Work out the finished part from the listing and answer in its coordinate system (mm). Give positions to 0.01 mm unless a question says otherwise; leave off trailing zeros. Write each loop counter-clockwise with the first axis right and the second up, starting at its lowest first coordinate (ties: lowest second). Pieces come first, ordered by that corner, then holes.
1) Find section B-B (x = -4). Determine the outline of the cut face in (y, z), plus the area to 3 significant figures.
2) Straight lines are drawn through the part: probe 1 along Y at (x, z) = (-60, 46.45); probe 2 along X at (y, z) = (12.75, -47); probe 3 along Z at (x, y) = (-49, 6.75). For each, find the intervals that lie inside material, in ascending order.
3) Find section C-C (z = -20). Determine the outline of the cut face in (x, y).
4) Find section D-D (y = 8.09). Determine the outline of the cut face in (x, z), plus the area to 3 significant figures.
5) Find section A-A (y = 16.5). Determine the outline of the cut face in (x, z), plus the area to 3 significant figures.
6) Given pin 1 Ø6 at (x, y) = (60, 2.5) entering from +Z; pin 2 Ø2 at (y, z) = (21.5, -49) entering from -X; pin 3 Ø2.5 at (x, z) = (-59, 46) entering from +Y; pin 4 Ø10 at (x, y) = (55.5, 24.5) entering from +Z, each flat-ended and moving along its own axis, determine where each tip first touches the part or whether it passes through.
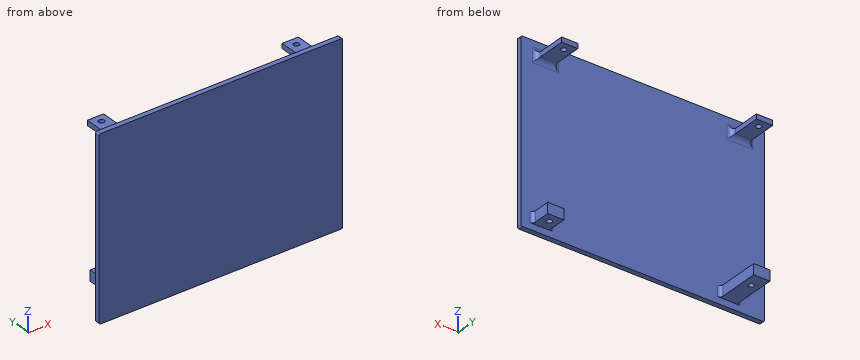
```python
from build123d import *

# Parameters (mm, degrees)
SKETCH1_W            = 150
SKETCH1_H            = 110
BOSS_EXTRUDE1_DEPTH  = 1.5
SKETCH2_W            = 10
SKETCH2_H            = 6.5
BOSS_EXTRUDE2_DEPTH  = 12
SKETCH3_W            = 10
SKETCH3_H            = 6.5
BOSS_EXTRUDE3_DEPTH  = 15
M3_CLEARANCE_HOLE1_D = 3.4
FILLET1_R            = 2
M3_CLEARANCE_HOLE2_D = 3.4
SKETCH8_W            = 10
SKETCH8_H            = 3
BOSS_EXTRUDE4_DEPTH  = 20
FILLET2_R            = 3
M3_CLEARANCE_HOLE3_D = 3.4
FILLET2_OF_MIRROR1_R = 3
FILLET3_R            = 1


with BuildPart() as part:
    # Sketch1 → Boss-Extrude1 (new, symmetric)
    with BuildSketch(Plane(origin=(0, 0, 0), x_dir=(1, 0, 0), z_dir=(0, 1, 0))):
        Rectangle(SKETCH1_W, SKETCH1_H)
    extrude(amount=BOSS_EXTRUDE1_DEPTH, both=True)

    # Sketch2 → Boss-Extrude2 (add)
    with BuildSketch(Plane(origin=(0, 1.5, 0), x_dir=(1, 0, 0), z_dir=(0, 1, 0))):
        with Locations((62.57, 47.75)):
            Rectangle(SKETCH2_W, SKETCH2_H)
        with Locations((-53, 47.75)):
            Rectangle(SKETCH2_W, SKETCH2_H)
    extrude(amount=BOSS_EXTRUDE2_DEPTH)

    # Sketch3 → Boss-Extrude3 (add)
    with BuildSketch(Plane(origin=(0, 13.5, 0), x_dir=(1, 0, 0), z_dir=(0, 1, 0))):
        with Locations((-53, 47.75)):
            Rectangle(SKETCH3_W, SKETCH3_H)
    extrude(amount=BOSS_EXTRUDE3_DEPTH)

    # M3 Clearance Hole1 (through all)
    with Locations(Plane.XY.offset(-44.5)):
        with Locations((-53, 19.77)):
            Hole(M3_CLEARANCE_HOLE1_D / 2)

    # Fillet1
    fillet1_edges = [part.edges().sort_by_distance(p)[0] for p in [
        (67.57, 1.5, -47.75),
        (57.57, 1.5, -47.75),
        (-48, 1.5, -47.75),
        (-58, 1.5, -47.75),
    ]]
    fillet(fillet1_edges, radius=FILLET1_R)

    # M3 Clearance Hole2 (through all)
    with Locations(Plane.XY.offset(-44.5)):
        with Locations((62.57, 8.09)):
            Hole(M3_CLEARANCE_HOLE2_D / 2)

    # Sketch8 → Boss-Extrude4 (add)
    with BuildSketch(Plane(origin=(0, 1.5, 0), x_dir=(1, 0, 0), z_dir=(0, 1, 0))):
        with Locations((-60, -46.5)):
            Rectangle(SKETCH8_W, SKETCH8_H)
    boss_extrude4 = extrude(amount=BOSS_EXTRUDE4_DEPTH)

    # Fillet2
    fillet2_edges = [part.edges().sort_by_distance(p)[0] for p in [
        (-55, 1.5, 46.5),
        (-60, 1.5, 45),
        (-65, 1.5, 46.5),
        (-60, 1.5, 48),
    ]]
    fillet(fillet2_edges, radius=FILLET2_R)

    # M3 Clearance Hole3 (through all)
    with Locations(Plane.XY.offset(48)):
        with Locations((-60, 16.5)):
            m3_clearance_hole3 = Hole(M3_CLEARANCE_HOLE3_D / 2)

    # Mirror1: Boss-Extrude4, M3 Clearance Hole3 across plane
    add(boss_extrude4.mirror(Plane(origin=(0, 0, 0), x_dir=(0, 0, 1), z_dir=(1, 0, 0))))
    add(m3_clearance_hole3.mirror(Plane(origin=(0, 0, 0), x_dir=(0, 0, 1), z_dir=(1, 0, 0))), mode=Mode.SUBTRACT)

    # Fillet2 of Mirror1
    fillet2_of_mirror1_edges = [part.edges().sort_by_distance(p)[0] for p in [
        (55, 1.5, 46.5),
        (60, 1.5, 45),
        (65, 1.5, 46.5),
        (60, 1.5, 48),
    ]]
    fillet(fillet2_of_mirror1_edges, radius=FILLET2_OF_MIRROR1_R)

    # Fillet3
    fillet3_edges = [part.edges().sort_by_distance(p)[0] for p in [
        (-75, 0, -55),
        (75, 0, -55),
        (75, 0, 55),
        (-75, 0, 55),
    ]]
    fillet(fillet3_edges, radius=FILLET3_R)


solid = part.part
```
Results:
1. outline: (-1.5, -55) - (1.5, -55) - (1.5, 55) - (-1.5, 55) - close
1. area: 330 mm2
2. probe 1: y = -1.5 to 14.8, 18.2 to 21.5
2. probe 2: x = -58 to -48, 57.57 to 67.57
2. probe 3: z = -51 to -44.5
3. outline: (-75, -1.5) - (75, -1.5) - (75, 1.5) - (-75, 1.5) - close
4. outline: (-65, 45) - (-55, 45) - (-55, 48) - (-65, 48) - close; (-58, -51) - (-48, -51) - (-48, -44.5) - (-58, -44.5) - close; (55, 45) - (65, 45) - (65, 48) - (55, 48) - close; (57.57, -51) - (60.87, -51) - (60.87, -44.5) - (57.57, -44.5) - close; (64.27, -51) - (67.57, -51) - (67.57, -44.5) - (64.27, -44.5) - close
4. area: 168 mm2
5. outline: (-65, 45) - (-61.7, 45) - (-61.7, 48) - (-65, 48) - close; (-58.3, 45) - (-55, 45) - (-55, 48) - (-58.3, 48) - close; (-58, -51) - (-48, -51) - (-48, -44.5) - (-58, -44.5) - close; (55, 45) - (58.3, 45) - (58.3, 48) - (55, 48) - close; (61.7, 45) - (65, 45) - (65, 48) - (61.7, 48) - close
5. area: 105 mm2
6. pin 1: stops at z = 55
6. pin 2: stops at x = -58
6. pin 3: stops at y = 21.5
6. pin 4: stops at z = 48
